For this review, take the finished solid that the model builds, in its own axes (mm). Face numbers are marked on the shaded views. A direction names the side the tool comes from. Round coordinates to 2 decimals unless told otherwise and drop trailing zeros. Write each loop counter-clockwise with the first axis right and the second up, starting at its lowest first coordinate (ties: lowest second). Pieces come first, ordered by that corner, then holes. Notation, with made-up numbers: (13, 37.5) -> (59, 37.5) arc R22 cw to (59, 70.5) -> close; hole circle Ø1 at (18.25, 54.25). An arc over 180 degrees is marked (long way). Write each question's results on one line, items separated by ' | '. Start each with the question number.
Item 1: To check wall thickness, follow line 1 along Y through (x, z) = (11, 1.75); line 2 along X through (y, z) = (1.25, 9.5); line 3 along Z through (x, y) = (43, 3). State the ranges of each line that lie inside material, in increasing order.
Item 2: Add section A-A (x = 3). State the section outline as (y, z) points (3 decimals).
Item 3: Tool access review of the marked faces 1 and 2: name each direction out of +Z, -Z, +X, -X, +Y, -Y from which nothing blocks a thin tool from reaching the whole face with its end or side.
Item 4: Add section D-D (x = 40). State the section outline as (y, z) points, plus the area to 3 significant figures.
Item 5: The part is to be moulded in two halves that separate along Y. For the marked faces 3, 4 and 5, say which applies: +Y half, -Y half, draft (parallel to the pull), parting line (faces both ways), or undercut.
Item 6: Add section B-B (z = 4). State the section outline as (x, y) points, plus the area to 3 significant figures.
Item 7: Add section C-C (y = 12.5). State the section outline as (x, z) points, plus the area to 3 significant figures.
Item 8: Clearance check with flat-ended pins moving along their axes: pin 1 (10 mm diameter, centred on x = 14, y = 14.5, fed in from +Z); pin 2 (0.8 mm diameter, centred on x = 26.5, y = 20.5, fed in from +Z); pin 3 (0.8 mm diameter, centred on y = 20.5, z = 11.5, fed in from -X) (3 decimals). State where each tip first meets the part, or that it passes through.
from build123d import *

# Parameters (mm, degrees)
BOX_W          = 50
BOX_H          = 20
BOX_DEPTH      = 12
THICKNESS_T    = 1
CYLINDER_R     = 8
CYLINDER_DEPTH = 1
BOX001_W       = 10
BOX001_H       = 22
BOX001_DEPTH   = 1
BOX002_W       = 8
BOX002_H       = 8
BOX002_DEPTH   = 1


with BuildPart() as part:
    # Box → Box (join)
    with BuildSketch(Plane.XY):
        with Locations((25, 10)):
            Rectangle(BOX_W, BOX_H)
    extrude(amount=BOX_DEPTH)

    # Thickness
    thickness_openings = [part.faces().sort_by_distance(p)[0] for p in [
        (25, 10, 12),
    ]]
    offset(amount=THICKNESS_T, openings=thickness_openings)

    # Cylinder → Cylinder (cut)
    with BuildSketch(Plane(origin=(8, 12, -1), x_dir=(1, 0, 0), z_dir=(0, 0, 1))):
        Circle(CYLINDER_R)
    extrude(amount=CYLINDER_DEPTH, mode=Mode.SUBTRACT)

    # Box001 → Box001 (cut)
    with BuildSketch(Plane(origin=(20, -1, 11), x_dir=(1, 0, 0), z_dir=(0, 0, 1))):
        with Locations((5, 11)):
            Rectangle(BOX001_W, BOX001_H)
    extrude(amount=BOX001_DEPTH, mode=Mode.SUBTRACT)

    # Box002 → Box002 (cut)
    with BuildSketch(Plane(origin=(0, 12, -1), x_dir=(1, 0, 0), z_dir=(0, 0, 1))):
        with Locations((4, 4)):
            Rectangle(BOX002_W, BOX002_H)
    extrude(amount=BOX002_DEPTH, mode=Mode.SUBTRACT)


solid = part.part
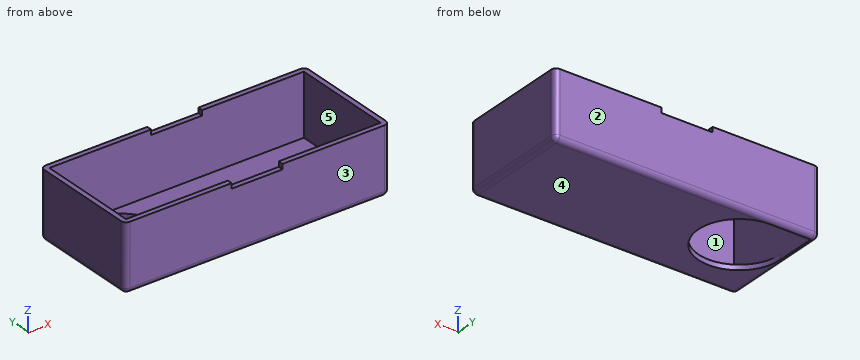
Responses:
1) line 1: y = -1 to 0, 20 to 21 | line 2: x = -1 to 0, 50 to 51 | line 3: z = -1 to 0
2) outline: (-1, 0) arc R1 ccw to (0, -1) -> (5.755, -1) -> (5.755, 0) -> (0, 0) -> (0, 12) -> (-1, 12) -> close; (20, -1) arc R1 ccw to (21, 0) -> (21, 12) -> (20, 12) -> close
3) face 1: +Z | face 2: +Z, -Z, +X, -X, +Y
4) outline: (-1, 0) arc R1 ccw to (0, -1) -> (20, -1) arc R1 ccw to (21, 0) -> (21, 12) -> (20, 12) -> (20, 0) -> (0, 0) -> (0, 12) -> (-1, 12) -> close | area: 45.6 mm^2
5) face 3: -Y half | face 4: draft | face 5: undercut
6) outline: (-1, 0) arc R1 ccw to (0, -1) -> (50, -1) arc R1 ccw to (51, 0) -> (51, 20) arc R1 ccw to (50, 21) -> (0, 21) arc R1 ccw to (-1, 20) -> close; hole (0, 0) -> (50, 0) -> (50, 20) -> (0, 20) -> close | area: 143 mm^2
7) outline: (-1, 0) arc R1 ccw to (0, -1) -> (0, 12) -> (-1, 12) -> close; (15.98, -1) -> (50, -1) arc R1 ccw to (51, 0) -> (51, 12) -> (50, 12) -> (50, 0) -> (15.98, 0) -> close | area: 59.6 mm^2
8) pin 1: stops at z = 0 | pin 2: stops at z = 11 | pin 3: stops at x = -0.995
